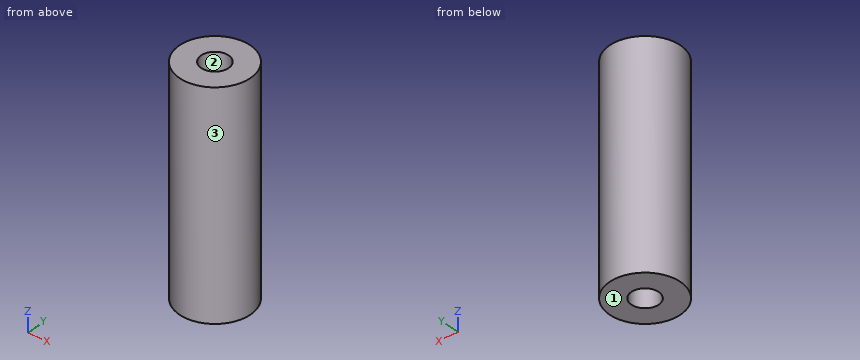
```python
from build123d import *

# Parameters (mm, degrees)
SKETCH1_R           = 16.4084
BOSS_EXTRUDE1_DEPTH = 101.6


with BuildPart() as part:
    # Sketch1 → Boss-Extrude1 (new body)
    with BuildSketch(Plane.XY):
        with Locations((-492.127121378, 1432.787310137)):
            Circle(SKETCH1_R)
    extrude(amount=BOSS_EXTRUDE1_DEPTH)

    # Sketch3 → Cut-Revolve1 (revolve, cut)
    with BuildSketch(Plane(origin=(-492.127121378, 0, 0), x_dir=(0, 0, -1), z_dir=(1, 0, 0))):
        Polygon((-91.44, 1445.385710137), (-10.16, 1445.385710137), (-10.16, 1439.137310137), (0, 1439.137310137), (0, 1432.787310137), (-101.6, 1432.787310137), (-101.6, 1439.137310137), (-91.44, 1439.137310137), align=None)
    revolve(axis=Axis((-492.127121378, 1432.787310137, 101.6), (0, 0, -1)), mode=Mode.SUBTRACT)


solid = part.part
```
For this review, take the finished solid that the model builds, in its own axes (mm). Face numbers are marked on the shaded views. Coordinates: 2 decimals unless noted, no trailing zeros. Loops run counter-clockwise (first coordinate to the right, second up) from the corner with the lowest first, then second, coordinate; pieces in that order, holes last. Notation, with made-up numbers: (2.25, 72) - (49.25, 72) arc R22 ccw to (49.25, 111) - close; hole circle Ø11 at (60, 34). An arc over 180 degrees is marked (long way). Use one line per item in the form item = value. Start each with the question number.
1) Take a section at A-A (x = -489). State the section outline as (y, z) points, plus the area to 3 significant figures.
2) Take a section at D-D (x = -501.5). State the section outline as (y, z) points.
3) Take a section at C-C (y = 1438). State the section outline as (x, z) points, plus the area to 3 significant figures.
4) To check wall thickness, follow probe 1 along Z at (x, y) = (-490.5, 1440); probe 2 along Y at (x, z) = (-497, 90); probe 3 along Y at (x, z) = (-492.5, 10). State the ranges of each line that lie inside material, in increasing order. Write a range as from..to.
5) Take a section at B-B (y = 1424.5). State the section outline as (x, z) points, plus the area to 3 significant figures.
6) Draft analysis for pull direction Y (two halves, no side actions). For the marked faces 1, 2 and 3, state which applies: released by +Y, released by -Y, zero draft, split by the parting line, or undercut.
7) For pin 1 (3 mm diameter, centred on x = -501, z = 66.5, fed in from -Y); pin 2 (12 mm diameter, centred on y = 1420, z = 68, fed in from +X); pin 3 (2 mm diameter, centred on y = 1445.5, z = 84.5, fed in from +X), all flat-tipped, find the tip position at first contact; note any pin that passes through.
From the geometry:
q1.outline = (1416.68, 0) - (1427.26, 0) - (1427.26, 10.16) - (1420.58, 10.16) - (1420.58, 91.44) - (1427.26, 91.44) - (1427.26, 101.6) - (1416.68, 101.6) - close; (1438.31, 0) - (1448.89, 0) - (1448.89, 101.6) - (1438.31, 101.6) - (1438.31, 91.44) - (1444.99, 91.44) - (1444.99, 10.16) - (1438.31, 10.16) - close
q1.area = 1,060 mm2
q2.outline = (1419.32, 0) - (1446.26, 0) - (1446.26, 101.6) - (1419.32, 101.6) - close; hole (1424.37, 10.16) - (1441.21, 10.16) - (1441.21, 91.44) - (1424.37, 91.44) - close
q3.outline = (-507.69, 0) - (-495.75, 0) - (-495.75, 10.16) - (-503.6, 10.16) - (-503.6, 91.44) - (-495.75, 91.44) - (-495.75, 101.6) - (-507.69, 101.6) - close; (-488.5, 0) - (-476.57, 0) - (-476.57, 101.6) - (-488.5, 101.6) - (-488.5, 91.44) - (-480.66, 91.44) - (-480.66, 10.16) - (-488.5, 10.16) - close
q3.area = 1,150 mm2
q4.probe_1 = 0..10.16, 91.44..101.6
q4.probe_2 = 1417.12..1421.17, 1444.41..1448.46
q4.probe_3 = 1416.38..1426.45, 1439.13..1449.19
q5.outline = (-506.29, 0) - (-477.97, 0) - (-477.97, 101.6) - (-506.29, 101.6) - close; hole (-501.62, 10.16) - (-482.64, 10.16) - (-482.64, 91.44) - (-501.62, 91.44) - close
q5.area = 1,340 mm2
q6.face_1 = zero draft
q6.face_2 = undercut
q6.face_3 = split by the parting line
q7.pin_1 = 1418.13
q7.pin_2 = -477.19
q7.pin_3 = -480.64
